```python
from build123d import *

# Parameters (mm, degrees)
EXTRUDE1_DEPTH = 1.397


with BuildPart() as part:
    # Sketch1 → Revolve1 (revolve)
    with BuildSketch(Plane.XY, mode=Mode.PRIVATE) as revolve1_sk:
        Polygon((0, 0), (0, -12.7), (1.203569231, -12.7), (1.4224, -12.481169231), (1.4224, -2.089184064), (2.7686, -0.540558115), (2.7686, 0), align=None)
    revolve(revolve1_sk.sketch.rotate(Axis((0, 0, 0), (0, -1, 0)), 90), axis=Axis((0, 0, 0), (0, -1, 0)))

    # Sketch2 → Extrude1 (cut)
    with BuildSketch(Plane(origin=(0, 0, 0), x_dir=(1, 0, 0), z_dir=(0, 1, 0))):
        Polygon((0, 0.909211204), (-0.7874, 0.454605602), (-0.7874, -0.454605602), (0, -0.909211204), (0.7874, -0.454605602), (0.7874, 0.454605602), align=None)
    extrude(amount=-EXTRUDE1_DEPTH, mode=Mode.SUBTRACT)


solid = part.part
```
The listing builds one solid part. Answer for the finished solid, in the listing's coordinates (mm). A direction names the side the tool comes from. Coordinates: 2 decimals unless noted, no trailing zeros. Loops run counter-clockwise (first coordinate to the right, second up) from the corner with the lowest first, then second, coordinate; pieces in that order, holes last. Notation, with made-up numbers: (1.25, -37) -> (19.25, -37) arc R23 cw to (19.25, -26) -> close; hole circle Ø5 at (-0.5, 6). An arc over 180 degrees is marked (long way). Use one line per item in the form item = value. Start each with the question number.
Item 1: The part is cut by section B-B on y = -11. Determine the outline of the cut face in (x, z), then the cut area to 3 significant figures.
Item 2: The part is cut by section A-A on z = 0. Determine the outline of the cut face in (x, y), then the cut area to 3 significant figures.
Item 3: A tool of negligible diameter and unlimited length cuts with its end or side. For faces 4 (the face through (0, -12.7, 0)), 5 (the face through (1.26, -7.21, 0.66)), 6 (the face through (0.787, -1, 0)), from which of +Z, -Z, +X, -X, +Y, -Y can it reach the whole face along a straight path? Write none if from no direction.
Item 4: The mould has two halves that part along Z. Classify faces 1 (the face through (0, -1.397, 0)), 2 (the face through (-0.83, -0.27, 2.64)), 3 (the face through (1, 0, 1)): released by +Z, released by -Z, zero draft, split by the parting line, or undercut.
Item 5: Flat-ended cylindrical pins translate along their axes: pin 1 Ø1 at (y, z) = (-3.5, -0.5) entering from -X; pin 2 Ø3 at (x, y) = (-1.5, -5.5) entering from -Z; pin 3 Ø0.5 at (x, z) = (0.5, 0.5) entering from +Y; pin 4 Ø2 at (y, z) = (-6.5, 2) entering from -X. Find the tip coordinate at first contact, or state that the pin passes through.
Item 6: The part is cut by section C-C on y = -1.75. Determine the outline of the cut face in (x, z).
Item 7: Consider L1, parallel to Y at x = 1.9, z = 1.5; L2, parallel to Z at x = 1, y = -10; L3, parallel to Z at x = 2.15, y = -0.75. Determine where each line is inside the solid, lowest interval first. Write a range as [from, to].
Answer key:
q1.outline = circle Ø2.84 at (0, 0)
q1.area = 6.36 mm2
q2.outline = (-2.77, -0.54) -> (-1.42, -2.09) -> (-1.42, -12.48) -> (-1.2, -12.7) -> (1.2, -12.7) -> (1.42, -12.48) -> (1.42, -2.09) -> (2.77, -0.54) -> (2.77, 0) -> (0.79, 0) -> (0.79, -1.4) -> (-0.79, -1.4) -> (-0.79, 0) -> (-2.77, 0) -> close
q2.area = 37.4 mm2
q3.face_4 = +Z, -Z, +X, -X, -Y
q3.face_5 = -Y
q3.face_6 = +Y
q4.face_1 = undercut
q4.face_2 = split by the parting line
q4.face_3 = zero draft
q5.pin_1 = -1.42
q5.pin_2 = -1.42
q5.pin_3 = 0
q5.pin_4 = -1.01
q6.outline = circle Ø3.43 at (0, 0)
q7.L1 = [-0.94, 0]
q7.L2 = [-1.01, 1.01]
q7.L3 = [-1.44, 1.44]
